Autodesk Inventor part; units mm, degrees
ref_plane "YZ Plane" through (0, 0, 0) normal (1, 0, 0) x (0, 1, 0)
ref_plane "XZ Plane" through (0, 0, 0) normal (0, 1, 0) x (-1, 0, 0)
ref_plane "XY Plane" through (0, 0, 0) normal (0, 0, 1) x (1, 0, 0)
sketch "Skizze1" plane through (0, 0, 0) normal (0, 0, 1) x (1, 0, 0)
  circle A0 centre (0, 0) radius 5
  dimension "d0" = 10
extrude "Extrusion1" add sketch "Skizze1" along normal mid plane 35
sketch "Skizze2" plane through (0, 0, 17.5) normal (0, 0, 1) x (1, 0, 0)
  circle A0 centre (0, 0) radius 5
sketch "Skizze3" plane through (0, 0, 0) normal (0, 1, 0) x (-1, 0, 0)
  circle A0 centre (0, 0) radius 5
  dimension "d3" = 10
extrude "Extrusion2" add sketch "Skizze3" along normal mid plane 35
sketch "Skizze4" plane through (0, 0, 0) normal (1, 0, 0) x (0, 1, 0)
  line L0 (0, 0) -> (5, -5)
  circle A0 centre (0, 0) radius 5
  dimension "d6" = 10
extrude "Extrusion3" add sketch "Skizze4" along normal mid plane 35
properties part number "DrehAchse"
CAD build for the part. Positions are in the model's coordinates, mm. A direction names the side the tool comes from. Give positions to 0.01 mm unless a question says otherwise; leave off trailing zeros. Loops run counter-clockwise (first coordinate to the right, second up) from the corner with the lowest first, then second, coordinate; pieces in that order, holes last. Notation, with made-up numbers: M 38.5,-5.75 L 62.5,-5.75 A29 cw 62.5,28.25 Z; hole C 72.25,-27 d7. An arc over 180 degrees is marked long. Use one line per item in the form item = value.
Item 1: Which spindle directions (+Z, -Z, +X, -X, +Y, -Y) get a long thin tool onto all of the face, cutting with end or side? Do faces 4 (the face through (5, -10, 0)), 5 (the face through (5, 10, 0)), 6 (the face through (10, -5, 0)), 7 (the face through (-5, 0, 10)). Say none if no direction does.
Determined:
face_4 = -Y
face_5 = +Y
face_6 = +X
face_7 = +Z
Item 2: Drill centre lines: probe 1 along Z at (x, y) = (0, 15.5); probe 2 along X at (y, z) = (13, 4); probe 3 along X at (y, z) = (5, 3.5). Where is each one in solid material? Low to high. Write a range as from..to.
Determined:
probe_1 = -5..5
probe_2 = -3..3
probe_3 = -3.57..3.57
Item 3: Slice it at C-C (y = 11.5). List the corners of the cut face in (x, z), plus the area to 3 significant figures.
Determined:
outline = C 0,0 d10
area = 78.5 mm2
Item 4: Slice it at A-A (x = 0). List the corners of the cut face in (y, z).
Determined:
outline = M -17.5,-5 L -5,-5 L -5,-17.5 L 5,-17.5 L 5,-5 L 17.5,-5 L 17.5,5 L 5,5 L 5,17.5 L -5,17.5 L -5,5 L -17.5,5 Z
Item 5: Two-plate mould, pull along Y, no slides. Class faces 1 (the face through (-5, 0, -10)), 2 (the face through (0, 0, -17.5)), 3 (the face through (0, -17.5, 0)): pulls with the +Y half, pulls with the -Y half, needs draft (parallel to the pull), parting line crosses it, or undercut.
Determined:
face_1 = parting line crosses it
face_2 = needs draft
face_3 = pulls with the -Y half
Item 6: Flat gauge pins, fed straight in: pin 1 (1.5 mm diameter, centred on x = 7.5, y = -12, fed in from +Z); pin 2 (5 mm diameter, centred on y = -14, z = 6, fed in from +X); pin 3 (12 mm diameter, centred on y = -13, z = 6.5, fed in from -X). Where does each tip first touch, or does it go through?
Determined:
pin_1 = through
pin_2 = 3.57
pin_3 = -4.97
